Geometry: see drawing. Coordinates: mm, zero at the bounding-box minimum. Give positions to 0.01 mm unless a question says otherwise; leave off trailing zeros. Loops run counter-clockwise (first coordinate to the right, second up) from the corner with the lowest first, then second, coordinate; pieces in that order, holes last. Notation, with made-up numbers: M 43.25,-23.5 L 85.25,-23.5 A18 ccw 85.25,-3.5 Z; hole C 13,32.5 d9. An arc over 180 degrees is marked long. Return JSON: item names as keys, results as strings. Group by question number.
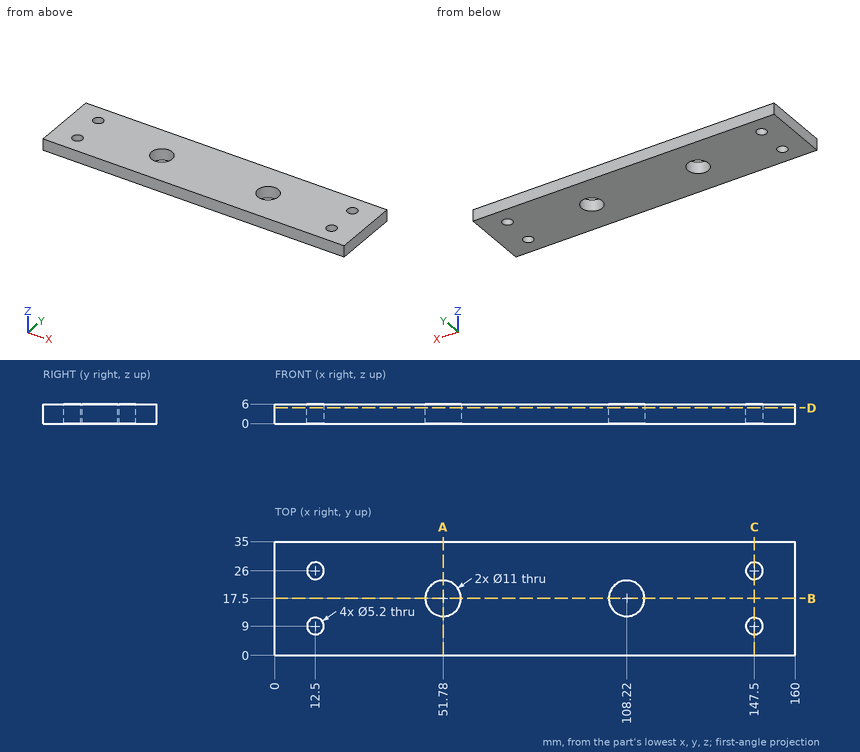
Item 1: Material intervals for line 1 (Y direction, x = 147.5, z = 3.8); line 2 (Y direction, x = 108.22, z = 3.9); line 3 (Y direction, x = 11, z = 5.55), sorted ascending. Write a range as from..to.
Item 2: Section A-A, the plane x = 51.78. Return loops of the section in (y, z).
Item 3: Section D-D, the plane z = 4.8. Return loops of the section in (x, y), then the cut area to 4 significant figures.
Item 4: Section B-B, the plane y = 17.5. Return loops of the section in (x, z), then the cut area to 3 significant figures.
Item 5: Section C-C, the plane x = 147.5. Return loops of the section in (y, z).
Answer below:
{
 "1": {"line 1": "0..6.4, 11.6..23.4, 28.6..35", "line 2": "0..12, 23..35", "line 3": "0..6.88, 11.12..23.88, 28.12..35"},
 "2": {"outline": "M 0,0 L 12,0 L 12,6 L 0,6 Z; M 23,0 L 35,0 L 35,6 L 23,6 Z"},
 "3": {"outline": "M 0,0 L 160,0 L 160,35 L 0,35 Z; hole C 12.5,9 d5.2; hole C 12.5,26 d5.2; hole C 51.78,17.5 d11; hole C 108.22,17.5 d11; hole C 147.5,9 d5.2; hole C 147.5,26 d5.2", "area": "5,325 mm^2"},
 "4": {"outline": "M 0,0 L 46.28,0 L 46.28,6 L 0,6 Z; M 57.28,0 L 102.72,0 L 102.72,6 L 57.28,6 Z; M 113.72,0 L 160,0 L 160,6 L 113.72,6 Z", "area": "828 mm^2"},
 "5": {"outline": "M 0,0 L 6.4,0 L 6.4,6 L 0,6 Z; M 11.6,0 L 23.4,0 L 23.4,6 L 11.6,6 Z; M 28.6,0 L 35,0 L 35,6 L 28.6,6 Z"}
}
